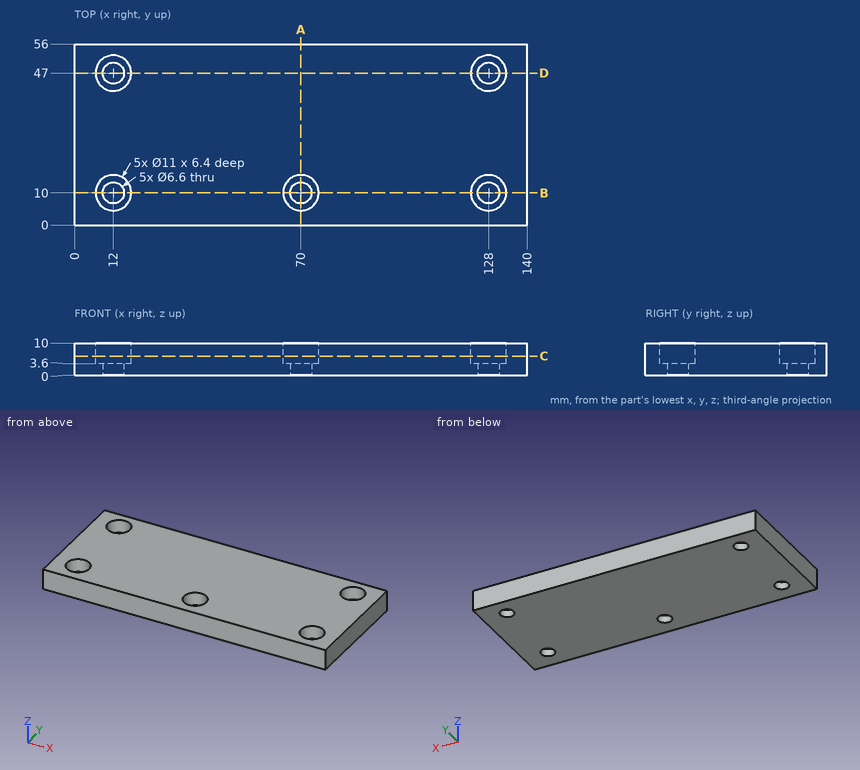
Check sheet for the drawn part. Datum: minimum x, y, z corner. Units: mm. Round coordinates to 2 decimals unless told otherwise and drop trailing zeros. Loops run counter-clockwise (first coordinate to the right, second up) from the corner with the lowest first, then second, coordinate; pieces in that order, holes last.
Item 1: Thickness scan on line 1 (Y direction, x = 128, z = 8.25); line 2 (Y direction, x = 12, z = 2); line 3 (X direction, y = 48.5, z = 8). Record the ranges inside material, lowest first.
Item 2: Cross-section at A-A on x = 70. Record the boundary of the cut face in (y, z), then the cut area to 3 significant figures.
Item 3: Cross-section at C-C on z = 6. Record the boundary of the cut face in (x, y).
Item 4: Gauge pin test, flat ends, axial feed: pin 1 (7.5 mm diameter, centred on x = 70, y = 10, fed in from +Z); pin 2 (6 mm diameter, centred on x = 128, y = 47, fed in from -Z). Record the tip position at first contact, or that the pin passes through.
Item 5: Cross-section at D-D on y = 47. Record the boundary of the cut face in (x, z).
Item 6: Cross-section at B-B on y = 10. Record the boundary of the cut face in (x, z).
Answer sheet:
1. line 1: y = 0 to 4.5, 15.5 to 41.5, 52.5 to 56
1. line 2: y = 0 to 6.7, 13.3 to 43.7, 50.3 to 56
1. line 3: x = 0 to 6.71, 17.29 to 122.71, 133.29 to 140
2. outline: (0, 0) - (6.7, 0) - (6.7, 3.6) - (4.5, 3.6) - (4.5, 10) - (0, 10) - close; (13.3, 0) - (56, 0) - (56, 10) - (15.5, 10) - (15.5, 3.6) - (13.3, 3.6) - close
2. area: 466 mm2
3. outline: (0, 0) - (140, 0) - (140, 56) - (0, 56) - close; hole circle Ø11 at (12, 10); hole circle Ø11 at (12, 47); hole circle Ø11 at (70, 10); hole circle Ø11 at (128, 10); hole circle Ø11 at (128, 47)
4. pin 1: stops at z = 3.6
4. pin 2: passes through
5. outline: (0, 0) - (8.7, 0) - (8.7, 3.6) - (6.5, 3.6) - (6.5, 10) - (0, 10) - close; (15.3, 0) - (124.7, 0) - (124.7, 3.6) - (122.5, 3.6) - (122.5, 10) - (17.5, 10) - (17.5, 3.6) - (15.3, 3.6) - close; (131.3, 0) - (140, 0) - (140, 10) - (133.5, 10) - (133.5, 3.6) - (131.3, 3.6) - close
6. outline: (0, 0) - (8.7, 0) - (8.7, 3.6) - (6.5, 3.6) - (6.5, 10) - (0, 10) - close; (15.3, 0) - (66.7, 0) - (66.7, 3.6) - (64.5, 3.6) - (64.5, 10) - (17.5, 10) - (17.5, 3.6) - (15.3, 3.6) - close; (73.3, 0) - (124.7, 0) - (124.7, 3.6) - (122.5, 3.6) - (122.5, 10) - (75.5, 10) - (75.5, 3.6) - (73.3, 3.6) - close; (131.3, 0) - (140, 0) - (140, 10) - (133.5, 10) - (133.5, 3.6) - (131.3, 3.6) - close
